```python
from build123d import *

# Parameters (mm, degrees)
SKETCH017_R             = 1.6
PAD008_DEPTH            = 4.95
SKETCH018_R             = 7.5
PAD009_DEPTH            = 15
SKETCH019_R             = 5.55
POCKET004_DEPTH         = 14
BODY004_PLACEMENT_ANGLE = 90


with BuildPart() as part:
    # Sketch017 (on DatumPlane) → Pad008 (new body, symmetric)
    with BuildSketch(Plane(origin=(110, 5, 25), x_dir=(0, 0, 1), z_dir=(0, -1, 0))):
        with BuildLine():
            ThreePointArc((8, -2.2e-05), (0, 8), (-8, -2.2e-05))
            Line((-7, -6.742665), (-8, -2.2e-05))
            Line((-7, -9.356116), (-7, -6.742665))
            Line((7, -9.356116), (-7, -9.356116))
            Line((7, -6.742665), (7, -9.356116))
            Line((8, -2.2e-05), (7, -6.742665))
        make_face()
        Circle(SKETCH017_R, mode=Mode.SUBTRACT)
    extrude(amount=PAD008_DEPTH, both=True)

    # Sketch018 (on DatumPlane) → Pad009 (join)
    with BuildSketch(Plane(origin=(119.356116, 5, 25), x_dir=(0, 0, 1), z_dir=(1, 0, 0))):
        Circle(SKETCH018_R)
    extrude(amount=PAD009_DEPTH)

    # Sketch019 (on DatumPlane) → Pocket004 (cut)
    with BuildSketch(Plane(origin=(134.356116, 5, 25), x_dir=(0, 0, 1), z_dir=(1, 0, 0))):
        Circle(SKETCH019_R)
    extrude(amount=-POCKET004_DEPTH, mode=Mode.SUBTRACT)


with BuildPart() as part_1:
    # Body004 placement: moved
    add(part.part.moved(Location((35, 0, 71))).rotate(Axis((35, 0, 71), (0, 1, 0)), BODY004_PLACEMENT_ANGLE))


solid = part_1.part
```
Source: CAD feature listing. Evaluate the final solid. Frame: model axes, mm. A direction names the side the tool comes from. Round coordinates to 2 decimals unless told otherwise and drop trailing zeros. Loops run counter-clockwise (first coordinate to the right, second up) from the corner with the lowest first, then second, coordinate; pieces in that order, holes last. Notation, with made-up numbers: M 2,50 L 33,50 A29 ccw 33,75 Z; hole C 8.25,33 d1. An arc over 180 degrees is marked long. Use a Markdown table: item, result. Add a question column.
1. Set-up query: faces 4 (the flat face through (60, 11, -48.356)), 5 (the flat face through (60, 5, -49.356)), 6 (the flat face through (60, -1, -48.356)), 7 (the flat face through (67.507, 4.931, -42.324)). Return all of +Z, -Z, +X, -X, +Y, -Y with unobstructed straight access to the full face (end or side cutting, diameter ignored); none if empty.
2. Pull-direction query (X, two-part tool) for faces 1 (the flat face through (53, 5, -47)), 2 (the cylindrical face through (52.507, 4.67, -55.751)), 3 (the cylindrical face through (54.455, 4.756, -56.454)); classes: +X half, -X half, draft (parallel to the pull), parting line (faces both ways), or undercut.
3. Contact query for flat-ended pins moving along their axis: pin 1 (1.1 mm diameter, centred on x = 53.5, y = 1, fed in from -Z); pin 2 (0.8 mm diameter, centred on y = 3.5, z = -46.5, fed in from +X); pin 3 (0.8 mm diameter, centred on x = 59, y = -1, fed in from +Z); pin 4 (3 mm diameter, centred on x = 62.5, z = -40.5, fed in from +Y). Output: stop coordinate, or through.
4. Cut plane D-D, the plane x = 57.25. Output: boundary loops of the cut face in (y, z), and give its area (3 significant figures).
5. Ray query, line 1 along Z through (x, y) = (60, 4); line 2 along X through (y, z) = (5, -56.5); line 3 along Y through (x, z) = (60, -58). Return the intervals inside material, ascending. Write a range as [from, to].
6. Cut plane C-C, the plane z = -54. Output: boundary loops of the cut face in (x, y), and give its area (3 significant figures).
7. Cut plane B-B, the plane y = 5. Output: boundary loops of the cut face in (x, z), and give its area (3 significant figures).
8. Cut plane A-A, the plane x = 60. Output: boundary loops of the cut face in (y, z).
Solution:
| question | item | result |
|---|---|---|
| 1 | face 4 | +Z, +X, -X, +Y |
| 1 | face 5 | -Z |
| 1 | face 6 | +Z, +X, -X, -Y |
| 1 | face 7 | +X, +Y, -Y |
| 2 | face 1 | -X half |
| 2 | face 2 | parting line |
| 2 | face 3 | undercut |
| 3 | pin 1 | stops at z = -63.36 |
| 3 | pin 2 | stops at x = 67 |
| 3 | pin 3 | stops at z = -48.36 |
| 3 | pin 4 | stops at y = 9.95 |
| 4 | outline | M -1.98,-63.36 L 0.18,-63.36 L 0.18,-49.36 L 9.82,-49.36 L 9.82,-63.36 L 11.98,-63.36 L 11.98,-48.36 L 9.95,-48.36 L 9.95,-31.49 L 0.05,-31.49 L 0.05,-48.36 L -1.98,-48.36 Z |
| 4 | area | 241 mm2 |
| 5 | line 1 | z = [-49.36, -40.6], [-37.4, -31] |
| 5 | line 2 | x = [52.5, 54.45], [65.55, 67.5] |
| 5 | line 3 | y = [-2.5, -0.55], [10.55, 12.5] |
| 6 | outline | C 60,5 d15; hole C 60,5 d11.1 |
| 6 | area | 79.9 mm2 |
| 7 | outline | M 52,-39 L 53,-45.74 L 53,-48.36 L 52.5,-48.36 L 52.5,-63.36 L 54.45,-63.36 L 54.45,-49.36 L 65.55,-49.36 L 65.55,-63.36 L 67.5,-63.36 L 67.5,-48.36 L 67,-48.36 L 67,-45.74 L 68,-39 A8 ccw Z; hole C 60,-39 d3.2 |
| 7 | area | 300 mm2 |
| 8 | outline | M -2.5,-63.36 L -0.55,-63.36 L -0.55,-49.36 L 10.55,-49.36 L 10.55,-63.36 L 12.5,-63.36 L 12.5,-48.36 L 9.95,-48.36 L 9.95,-40.6 L 0.05,-40.6 L 0.05,-48.36 L -2.5,-48.36 Z; M 0.05,-37.4 L 9.95,-37.4 L 9.95,-31 L 0.05,-31 Z |
